Autodesk Inventor part; units mm, degrees
ref_plane "YZ Plane" through (0, 0, 0) normal (1, 0, 0) x (0, 1, 0)
ref_plane "XZ Plane" through (0, 0, 0) normal (0, 1, 0) x (-1, 0, 0)
ref_plane "XY Plane" through (0, 0, 0) normal (0, 0, 1) x (1, 0, 0)
sketch "Sketch5" plane through (0, 0, 0) normal (0, 0, 1) x (1, 0, 0)
  line L0 (-11.1597, 4.6835) -> (8.8403, 4.6835)
  line L1 (8.8403, 4.6835) -> (8.8403, -15.3165)
  line L2 (8.8403, -15.3165) -> (-11.1597, -15.3165)
  line L3 (-11.1597, -15.3165) -> (-11.1597, 4.6835)
  point P0 (0, 0)
  dimension "d13" = 20
  dimension "d14" = 20
extrude "Extrusion5" add sketch "Sketch5" along normal blind 8
sketch "Sketch6" plane through (0, 0, 8) normal (0, 0, 1) x (1, 0, 0)
  line L0 (-10.6667, 4.1905) -> (8.3333, 4.1905)
  line L1 (8.3333, 4.1905) -> (8.3333, -14.8095)
  line L2 (8.3333, -14.8095) -> (-10.6667, -14.8095)
  line L3 (-10.6667, -14.8095) -> (-10.6667, 4.1905)
  point P0 (0, 0)
  dimension "d17" = 19
  dimension "d18" = 19
extrude "Extrusion6" cut sketch "Sketch6" against normal blind 7
sketch "Sketch11" plane through (8.8403, -15.3165, 0) normal (1, 0, 0) x (0, 0, -1)
  line L0 (-4.9297, 9.3778) -> (-2.9693, 9.3778)
  line L1 (-2.9693, 9.3778) -> (-2.9693, 11.3958)
  line L2 (-2.9693, 11.3958) -> (-4.9297, 11.3958)
  line L3 (-4.9297, 11.3958) -> (-4.9297, 9.3778)
  point P0 (0, 15.3165)
extrude "Extrusion11" add sketch "Sketch11" along normal blind 30
sketch "Sketch12" plane through (8.8403, -5.9387, 2.9693) normal (0, -1, 0) x (1, 0, 0)
  circle A0 centre (26.9647, 0.9802) radius 0.3
  point P0 (-8.8403, -2.9693)
  dimension "d35" = 0.6
extrude "Extrusion12" cut sketch "Sketch12" against normal blind 30
sketch "Sketch13" plane through (0, 0, 0) normal (0, 0, -1) x (-1, 0, 0)
  line L0 (-9, 6.898) -> (15, 6.898)
  line L1 (15, 6.898) -> (15, -17.102)
  line L2 (15, -17.102) -> (-9, -17.102)
  line L3 (-9, -17.102) -> (-9, 6.898)
  point P0 (0, 0)
  dimension "d38" = 24
  dimension "d39" = 24
extrude "Extrusion13" cut sketch "Sketch13" against normal blind 10
sketch "Sketch14" plane through (9, -5.9387, 4.9297) normal (-1, 0, 0) x (0, 0, 1)
  line L0 (-1.9603, 0) -> (-1.9603, 2.018)
  line L1 (-1.9603, -10.5808) -> (8.0397, -10.5808)
  line L2 (8.0397, -10.5808) -> (8.0397, 13.4192)
  line L3 (8.0397, 13.4192) -> (-1.9603, 13.4192)
  line L4 (-1.9603, 13.4192) -> (-1.9603, -10.5808)
  point P0 (-4.9297, 5.9387)
  dimension "d42" = 10
  dimension "d43" = 24
extrude "Extrusion14" add sketch "Sketch14" along normal blind 24
sketch "Sketch15" plane through (9, -16.5195, 12.9693) normal (0, 0, 1) x (1, 0, 0)
  line L0 (-1.5875, 22.225) -> (-22.225, 22.225)
  line L1 (-22.225, 22.225) -> (-22.225, 1.5875)
  line L2 (-22.225, 1.5875) -> (-1.5875, 1.5875)
  line L3 (-1.5875, 1.5875) -> (-1.5875, 22.225)
  point P0 (-9, 16.5195)
extrude "Extrusion15" cut sketch "Sketch15" against normal blind 8
sketch "Sketch16" plane through (9, -5.9387, 4.9297) normal (1, 0, 0) x (0, 0, -1)
  line L0 (1.9603, 13.4192) -> (1.9603, -10.5808)
  line L1 (1.9603, 7.9375) -> (-1.5875, 7.9375)
  line L2 (-1.5875, 7.9375) -> (-1.5875, -4.7625)
  line L3 (-1.5875, -4.7625) -> (1.9603, -4.7625)
  line L4 (1.9603, -4.7625) -> (1.9603, 7.9375)
  point P0 (4.9297, 5.9387)
  point P1 (1.9603, -4.7625)
extrude "Extrusion16" add sketch "Sketch16" along normal blind 2
properties part number "pusher"
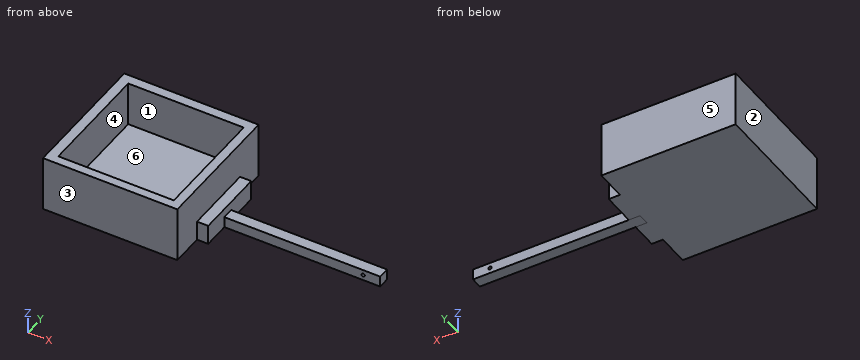
Read the model definition and answer for the solid it produces. Units are mm, in the model's axes. Face numbers are marked on the shaded views. A direction names the side the tool comes from. Round coordinates to 2 decimals unless told otherwise and drop trailing zeros. Order: outer loops, then holes, each group sorted by start corner. A loop starts at its lowest first (then second) coordinate and runs counter-clockwise, first axis right, second up.
1) The part is cut by section A-A on z = 5.5. Write down the section's boundary in (x, y) (1 decimal).
2) The part is cut by section B-B on x = 4. Write down the section's boundary in (y, z), plus the area to 3 significant figures.
3) Straight lines are drawn through the part: L1, parallel to Y at x = -2.5, z = 6; L2, parallel to X at y = -11.5, z = 6.25 (1 decimal); L3, parallel to X at y = -9.75, z = 5.25 (1 decimal). For each, find the intervals that lie inside material, in ascending order.
4) The part is cut by section D-D on z = 9. Write down the section's boundary in (x, y) (1 decimal).
5) The mould has two halves that part along X. Classify the marked faces 1, 2, 3 and 4: released by +X, released by -X, zero draft, split by the parting line, or undercut.
6) The part is cut by section C-C on y = -11.75. Write down the section's boundary in (x, z) (1 decimal), plus the area to 3 significant figures.
7) Flat-ended cylindrical pins translate along their axes: pin 1 (1 mm diameter, centred on x = 23, z = 4, fed in from -Y); pin 2 (1.6 mm diameter, centred on x = 10, z = 4.5, fed in from +Y); pin 3 (1.6 mm diameter, centred on x = 24, z = 4, fed in from +Y). Find the tip coordinate at first contact, or state that the pin passes through.
8) For the marked faces 5 and 6, determine the directions among +Z, -Z, +X, -X, +Y, -Y from which every point of the face is accessible in a straight line to the end or side of a thin tool.
Resolved:
1. outline: (-15, -16.5) - (9, -16.5) - (9, -10.7) - (11, -10.7) - (11, 2) - (9, 2) - (9, 7.5) - (-15, 7.5) - close; hole (-13.2, -14.9) - (7.4, -14.9) - (7.4, 5.7) - (-13.2, 5.7) - close
2. outline: (-16.52, 2.97) - (7.48, 2.97) - (7.48, 12.97) - (5.71, 12.97) - (5.71, 4.97) - (-14.93, 4.97) - (-14.93, 12.97) - (-16.52, 12.97) - close
2. area: 74.9 mm2
3. L1: y = -16.52 to -14.93, 5.71 to 7.48
3. L2: x = -15 to -13.2, 7.4 to 9
3. L3: x = -15 to -13.2, 7.4 to 11
4. outline: (-15, -16.5) - (9, -16.5) - (9, 7.5) - (-15, 7.5) - close; hole (-13.2, -14.9) - (7.4, -14.9) - (7.4, 5.7) - (-13.2, 5.7) - close
5. face 1: undercut
5. face 2: released by -X
5. face 3: zero draft
5. face 4: undercut
6. outline: (-15, 3) - (9, 3) - (9, 13) - (7.4, 13) - (7.4, 5) - (-13.2, 5) - (-13.2, 13) - (-15, 13) - close
6. area: 74.9 mm2
7. pin 1: stops at y = -5.94
7. pin 2: stops at y = 2
7. pin 3: stops at y = -3.92
8. face 5: +Z, -Z, +X, -X, +Y
8. face 6: +Z
